from build123d import *

# Parameters (mm, degrees)
BOSS_EXTRUDE1_DEPTH = 23
FILLET1_R           = 0.3


with BuildPart() as part:
    # Sketch1 → Boss-Extrude1 (new body)
    with BuildSketch(Plane(origin=(0, 0, 0), x_dir=(1, 0, 0), z_dir=(0, 1, 0))):
        Polygon((0.8, 0.8), (2.3, 0.8), (2.3, -0.8), (0.8, -0.8), (0.8, -2.3), (-0.8, -2.3), (-0.8, -0.8), (-2.3, -0.8), (-2.3, 0.8), (-0.8, 0.8), (-0.8, 2.3), (0.8, 2.3), align=None)
    extrude(amount=BOSS_EXTRUDE1_DEPTH)

    # Fillet1
    fillet1_edges = [part.edges().sort_by_distance(p)[0] for p in [
        (1.55, 0, 0.8),
        (0.8, 0, 1.55),
        (0.8, 23, -1.55),
        (0, 0, 2.3),
        (-0.8, 0, 1.55),
        (-1.55, 0, 0.8),
        (-2.3, 0, 0),
        (-1.55, 0, -0.8),
        (-0.8, 0, -1.55),
        (0, 0, -2.3),
        (0.8, 0, -1.55),
        (1.55, 0, -0.8),
        (2.3, 0, 0),
        (0, 23, -2.3),
        (-0.8, 23, -1.55),
        (-1.55, 23, -0.8),
        (-2.3, 23, 0),
        (-1.55, 23, 0.8),
        (-0.8, 23, 1.55),
        (0, 23, 2.3),
        (0.8, 23, 1.55),
        (1.55, 23, 0.8),
        (2.3, 23, 0),
        (1.55, 23, -0.8),
    ]]
    fillet(fillet1_edges, radius=FILLET1_R)


solid = part.part
Geometry check sheet. Reference: the model listing, model coordinates, mm. A direction names the side the tool comes from. Coordinates: 2 decimals unless noted, no trailing zeros. Order: outer loops, then holes, each group sorted by start corner. A loop starts at its lowest first (then second) coordinate and runs counter-clockwise, first axis right, second up. Notation, with made-up numbers: (70, 18) -> (102, 18) arc R22 ccw to (102, 35) -> close; hole circle Ø10 at (17.25, -28.75). An arc over 180 degrees is marked (long way). Use a Markdown table: item, result. Add a question column.
1. Go/stop test with flat-tipped pins: pin 1 Ø1.2 at (y, z) = (13, -2) entering from -X; pin 2 Ø0.7 at (y, z) = (8, -2) entering from +X. Record where each tip stops, or that it passes through.
2. Material ranges on L1, parallel to X at y = 10.25, z = -1.6; L2, parallel to Y at x = -0.7, z = 1.15, recorded low to high.
3. Cross-section at B-B (y = 17). Enter the section's corners in (x, z), and give its area (3 significant figures).
4. Cross-section at A-A (x = -1.15). Enter the section's corners in (y, z).
5. Set-up check for faces 1 (the face through (0, 11, -2.3)), 2 (the face through (-2, 11, -0.8)), 3 (the face through (2, 11, -0.8)), 4 (the face through (0.8, 11, 2)), 5 (the face through (-0.8, 11, 2)): record each of +Z, -Z, +X, -X, +Y, -Y from which the full face is reachable in a straight line by a thin tool's end or side.
Filled sheet:
| question | item | result |
|---|---|---|
| 1 | pin 1 | x = -0.8 |
| 1 | pin 2 | x = 0.8 |
| 2 | L1 | -0.8 to 0.8 |
| 2 | L2 | 0.08 to 22.92 |
| 3 | outline | (-2.3, -0.8) -> (-0.8, -0.8) -> (-0.8, -2.3) -> (0.8, -2.3) -> (0.8, -0.8) -> (2.3, -0.8) -> (2.3, 0.8) -> (0.8, 0.8) -> (0.8, 2.3) -> (-0.8, 2.3) -> (-0.8, 0.8) -> (-2.3, 0.8) -> close |
| 3 | area | 12.2 mm2 |
| 4 | outline | (0, -0.5) arc R0.3 ccw to (0.3, -0.8) -> (22.7, -0.8) arc R0.3 ccw to (23, -0.5) -> (23, 0.5) arc R0.3 ccw to (22.7, 0.8) -> (0.3, 0.8) arc R0.3 ccw to (0, 0.5) -> close |
| 5 | face 1 | -Z, +X, -X, +Y, -Y |
| 5 | face 2 | -Z, -X, +Y, -Y |
| 5 | face 3 | -Z, +X, +Y, -Y |
| 5 | face 4 | +Z, +X, +Y, -Y |
| 5 | face 5 | +Z, -X, +Y, -Y |
